```python
from build123d import *

# Parameters (mm, degrees)
SKETCH_2_R      = 2.1
SKETCH_2_R_2    = 1.6
SKETCH_2_R_3    = 8
SKETCH_2_R_4    = 31
EXTRUDE_1_DEPTH = 10


with BuildPart() as part:
    # 草图2 → 凸台-拉伸1 (new body)
    with BuildSketch(Plane.XY):
        with BuildLine():
            Line((81.141158551, 103.50108814), (-37.710043915, 21.419438295))
            Line((-37.710043915, 21.419438295), (-82.77215927, -13.299292234))
            ThreePointArc((-82.77215927, -13.299292234), (-93.160663011, -93.428150421), (-13.031804825, -83.03964668))
            Line((-13.031804825, -83.03964668), (21.686925704, -37.977531325))
            Line((21.686925704, -37.977531325), (33.707740984, 0.91334164))
            Line((33.707740984, 0.91334164), (103.768575549, 80.873671142))
            ThreePointArc((103.768575549, 80.873671142), (103.768575549, 103.50108814), (81.141158551, 103.50108814))
        make_face()
        with Locations((17.176075274, -35.63988511)):
            Circle(SKETCH_2_R, mode=Mode.SUBTRACT)
        with Locations((67.37860693, 69.690245447)):
            Circle(SKETCH_2_R, mode=Mode.SUBTRACT)
        with Locations((40.414990788, 69.298046443)):
            Circle(SKETCH_2_R, mode=Mode.SUBTRACT)
        with Locations((15.729805139, 52.249832182)):
            Circle(SKETCH_2_R, mode=Mode.SUBTRACT)
        with Locations((-8.95538051, 35.201617921)):
            Circle(SKETCH_2_R, mode=Mode.SUBTRACT)
        with Locations((29.24523113, 3.407383835)):
            Circle(SKETCH_2_R, mode=Mode.SUBTRACT)
        with Locations((49.015635424, 25.971317758)):
            Circle(SKETCH_2_R, mode=Mode.SUBTRACT)
        with Locations((66.149985812, 45.526727158)):
            Circle(SKETCH_2_R, mode=Mode.SUBTRACT)
        with Locations((-33.680842426, 18.211870041)):
            Circle(SKETCH_2_R, mode=Mode.SUBTRACT)
        with Locations((-105.098217171, -57.36570458)):
            Circle(SKETCH_2_R_2, mode=Mode.SUBTRACT)
        with Locations((-91.039342668, -23.424579083)):
            Circle(SKETCH_2_R_2, mode=Mode.SUBTRACT)
        with Locations((-57.098217171, -9.36570458)):
            Circle(SKETCH_2_R_2, mode=Mode.SUBTRACT)
        with Locations((-23.157091674, -23.424579083)):
            Circle(SKETCH_2_R_2, mode=Mode.SUBTRACT)
        with Locations((-9.098217171, -57.36570458)):
            Circle(SKETCH_2_R_2, mode=Mode.SUBTRACT)
        with Locations((-23.157091674, -91.306830077)):
            Circle(SKETCH_2_R_2, mode=Mode.SUBTRACT)
        with Locations((-57.098217171, -105.36570458)):
            Circle(SKETCH_2_R_2, mode=Mode.SUBTRACT)
        with Locations((-91.039342668, -91.306830077)):
            Circle(SKETCH_2_R_2, mode=Mode.SUBTRACT)
        with Locations((92.45486705, 92.187379641)):
            Circle(SKETCH_2_R_3, mode=Mode.SUBTRACT)
        with Locations((-100.110871654, -41.058909852)):
            Circle(SKETCH_2_R_2, mode=Mode.SUBTRACT)
        with Locations((-73.405011899, -100.378359063)):
            Circle(SKETCH_2_R_2, mode=Mode.SUBTRACT)
        with Locations((-14.085562688, -73.672499309)):
            Circle(SKETCH_2_R_2, mode=Mode.SUBTRACT)
        with Locations((-57.098217171, -57.36570458)):
            Circle(SKETCH_2_R_4, mode=Mode.SUBTRACT)
        with Locations((-15.153032377, -38.48181005)):
            Circle(SKETCH_2_R_2, mode=Mode.SUBTRACT)
        with Locations((-38.214322641, -99.310889374)):
            Circle(SKETCH_2_R_2, mode=Mode.SUBTRACT)
        with Locations((-99.043401964, -76.24959911)):
            Circle(SKETCH_2_R_2, mode=Mode.SUBTRACT)
        with Locations((-75.982111701, -15.420519787)):
            Circle(SKETCH_2_R_2, mode=Mode.SUBTRACT)
        with Locations((-40.791422442, -14.353050097)):
            Circle(SKETCH_2_R_2, mode=Mode.SUBTRACT)
    extrude(amount=EXTRUDE_1_DEPTH)


solid = part.part
```
The model under review builds one solid part; all positions refer to its coordinate system, in mm. Round coordinates to 2 decimals unless told otherwise and drop trailing zeros. Write each loop counter-clockwise with the first axis right and the second up, starting at its lowest first coordinate (ties: lowest second). Pieces come first, ordered by that corner, then holes. Notation, with made-up numbers: (14, -19.75) - (30, -19.75) arc R31 cw to (30, 16.25) - close; hole circle Ø1 at (25, -19). An arc over 180 degrees is marked (long way). Use one line per item in the form item = value.
Q1. For line 1 (Y direction, x = -42, z = 9.25); line 2 (X direction, y = -78, z = 6.75); line 3 (Y direction, x = 98.5, z = 4.25), list the stretches that pass through material, from the lowest coordinate up. Write a range as [from, to].
Answer key:
line_1 = [-106.08, -84.44], [-30.29, -15.4], [-13.3, 18.11]
line_2 = [-103.74, -80.23], [-33.96, -9.15]
line_3 = [74.86, 86.95], [97.43, 107]
Q2. Consider section A-A (z = 2.5). State how many separate pieces and enclosed holes the cut face has, and give its area (3 significant figures).
Answer key:
separate_pieces = 1
enclosed_holes = 27
area = 14,800 mm2
Q3. Insertion check: pin 1 Ø5 at (x, z) = (44.5, 2.5) entering from +Y; pin 2 Ø1 at (x, z) = (60, 2.5) entering from +Y; pin 3 Ø1.5 at (y, z) = (16, 6.5) entering from +X. Each pin has a flat end and moves straight along its axis. Give the tip position at first contact, or say it passes through.
Answer key:
pin_1 = 79.92
pin_2 = 89.25
pin_3 = 47.58
Q4. Consider section B-B (x = 1). State the section outline as (y, z) points, and give its area (3 significant figures).
Answer key:
outline = (-64.83, 0) - (48.15, 0) - (48.15, 10) - (-64.83, 10) - close
area = 1,130 mm2
Q5. Consider section C-C (y = 60). State the section outline as (x, z) points, and give its area (3 significant figures).
Answer key:
outline = (18.15, 0) - (85.48, 0) - (85.48, 10) - (18.15, 10) - close
area = 673 mm2
Q6. Draft analysis for pull direction X (two halves, no side actions). For faces 1 (the cylindrical face through (104.015, 103.25, 4.93)), 2 (the flat face through (68.248, 40.334, 4.93)), 3 (the cylindrical face through (86.106, 87.32, 4.93)), state which applies: +X half, -X half, draft (parallel to the pull), parting line (faces both ways), or undercut.
Answer key:
face_1 = parting line
face_2 = +X half
face_3 = undercut
